Source: CAD feature listing. Evaluate the final solid. Frame: model axes, mm. Face numbers are marked on the shaded views. A direction names the side the tool comes from. Round coordinates to 2 decimals unless told otherwise and drop trailing zeros. Loops run counter-clockwise (first coordinate to the right, second up) from the corner with the lowest first, then second, coordinate; pieces in that order, holes last. Notation, with made-up numbers: (34.5, -27.5) - (45.5, -27.5) arc R30 cw to (45.5, 2.5) - close; hole circle Ø7 at (62, -26). An arc over 180 degrees is marked (long way). Use CSV: the item, a comma, the result in double quotes. Start each with the question number.
from build123d import *

# Parameters (mm, degrees)
BASIC_SHAPE_SKETCH_W     = 18
BASIC_SHAPE_SKETCH_H     = 65
BASIC_SHAPE_DEPTH        = 2
CONNECTOR_SKETCH_W       = 7.4
CONNECTOR_SKETCH_H       = 8
CONNECTOR_DEPTH          = 7.25
CONNECTOR_HOLES_SKETCH_W = 3
CONNECTOR_HOLES_SKETCH_H = 4.5
CONNECTOR_HOLES_DEPTH    = 5
SKETCH1_W                = 18
SKETCH1_H                = 8
BOSS_EXTRUDE1_DEPTH      = 7.25


with BuildPart() as part:
    # Basic Shape Sketch → Basic Shape (new body)
    with BuildSketch(Plane.XY):
        Rectangle(BASIC_SHAPE_SKETCH_W, BASIC_SHAPE_SKETCH_H)
    extrude(amount=BASIC_SHAPE_DEPTH)

    # Connector Sketch → Connector (add)
    with BuildSketch(Plane(origin=(0, 0, 0), x_dir=(-1, 0, 0), z_dir=(0, 0, -1))):
        with Locations((0, -28.5)):
            Rectangle(CONNECTOR_SKETCH_W, CONNECTOR_SKETCH_H)
    extrude(amount=CONNECTOR_DEPTH)

    # Connector Holes Sketch → Connector Holes (cut)
    with BuildSketch(Plane.XZ.offset(32.5)):
        with Locations((-1.7, -3.5)):
            Rectangle(CONNECTOR_HOLES_SKETCH_W, CONNECTOR_HOLES_SKETCH_H)
        with Locations((1.7, -3.5)):
            Rectangle(CONNECTOR_HOLES_SKETCH_W, CONNECTOR_HOLES_SKETCH_H)
    extrude(amount=-CONNECTOR_HOLES_DEPTH, mode=Mode.SUBTRACT)

    # Sketch1 → Boss-Extrude1 (add)
    with BuildSketch(Plane(origin=(0, 0, 0), x_dir=(-1, 0, 0), z_dir=(0, 0, -1))):
        with Locations((0, 28.5)):
            Rectangle(SKETCH1_W, SKETCH1_H)
    extrude(amount=BOSS_EXTRUDE1_DEPTH)


solid = part.part
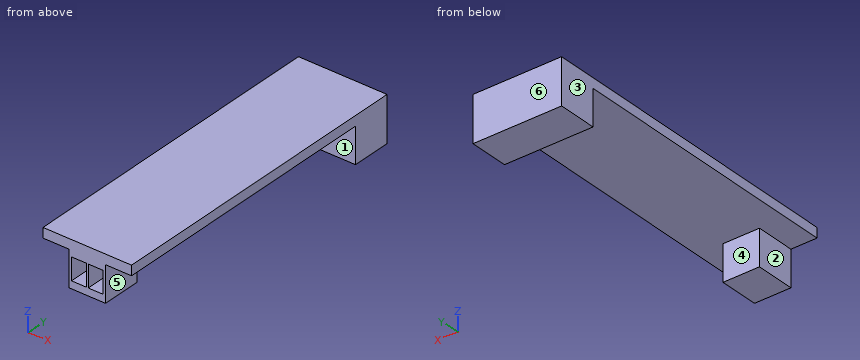
1. Reachability of the marked faces 1, 2 and 3 from +Z, -Z, +X, -X, +Y, -Y: full face, straight path, thin tool, end or side. Return the list, or none.
2. Section query B-B on x = -1.25. Return the cut outline in (y, z), and give its area (4 significant figures).
3. Mould query, pull axis Y, two halves, no side actions, for the marked faces 4, 5 and 6. Classes: +Y half, -Y half, draft (parallel to the pull), parting line (faces both ways), or undercut.
4. Section query A-A on z = -3.5. Return the cut outline in (x, y), and give its area (3 significant figures).
5. Line query: line 1 along Y through (x, z) = (0.25, -3.5); line 2 along Y through (x, z) = (1.5, -1); line 3 along Z through (x, y) = (-8, -21). Output: solid intervals per line, ascending.
6. Section query D-D on x = -6.75. Return the cut outline in (y, z), and give its area (3 significant figures).
7. Section query C-C on y = 14. Return the cut outline in (x, z), and give its area (3 significant figures).
8. Contact query for flat-ended pins moving along their axis: P1, Ø1, axis at x = -5, y = -8, coming from the -Z side; P2, Ø2, axis at y = -30.5, z = -3.5, coming from the +X side; P3, Ø2, axis at y = -27.5, z = -4, coming from the -X side. Output: stop coordinate, or through.
Values:
1,face 1,"-Z, +X, -X"
1,face 2,"-Z, -X, -Y"
1,face 3,"+Z, -Z, -X, +Y, -Y"
2,outline,"(-32.5, -7.25) - (-24.5, -7.25) - (-24.5, 0) - (24.5, 0) - (24.5, -7.25) - (32.5, -7.25) - (32.5, 2) - (-32.5, 2) - (-32.5, -1.25) - (-27.5, -1.25) - (-27.5, -5.75) - (-32.5, -5.75) - close"
2,area,"223.5 mm^2"
3,face 4,"undercut"
3,face 5,"draft"
3,face 6,"+Y half"
4,outline,"(-9, 24.5) - (9, 24.5) - (9, 32.5) - (-9, 32.5) - close; (-3.7, -32.5) - (-3.2, -32.5) - (-3.2, -27.5) - (-0.2, -27.5) - (-0.2, -32.5) - (0.2, -32.5) - (0.2, -27.5) - (3.2, -27.5) - (3.2, -32.5) - (3.7, -32.5) - (3.7, -24.5) - (-3.7, -24.5) - close"
4,area,"173 mm^2"
5,line 1,"y = -27.5 to -24.5, 24.5 to 32.5"
5,line 2,"y = -32.5 to -24.5, 24.5 to 32.5"
5,line 3,"z = 0 to 2"
6,outline,"(-32.5, 0) - (24.5, 0) - (24.5, -7.25) - (32.5, -7.25) - (32.5, 2) - (-32.5, 2) - close"
6,area,"188 mm^2"
7,outline,"(-9, 0) - (9, 0) - (9, 2) - (-9, 2) - close"
7,area,"36.0 mm^2"
8,P1,"stops at z = 0"
8,P2,"stops at x = 3.7"
8,P3,"stops at x = -3.7"
